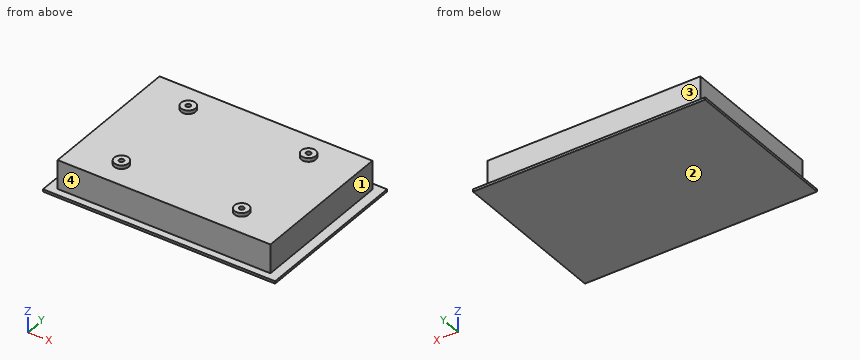
from build123d import *

# Parameters (mm, degrees)
SKETCH_1_W               = 193
SKETCH_1_H               = 134
EXTRUDE_1_DEPTH          = 2
SKETCH_2_W               = 177
SKETCH_2_H               = 122
EXTRUDE_2_DEPTH          = 24
CUT_EXTRUDE_1_DEPTH      = 10
CUT_EXTRUDE_1_DEPTH_BACK = 5
SKETCH_3_R               = 2
EXTRUDE_START            = 3
SKETCH_4_R               = 6
SKETCH_4_R_2             = 2
EXTRUDE_3_DEPTH          = 3


with BuildPart() as part:
    # 草图1 → 凸台-拉伸1 (new body)
    with BuildSketch(Plane.XY):
        Rectangle(SKETCH_1_W, SKETCH_1_H)
    extrude(amount=EXTRUDE_1_DEPTH)

    # 草图2 → 凸台-拉伸2 (add)
    with BuildSketch(Plane.XY.offset(2)):
        Rectangle(SKETCH_2_W, SKETCH_2_H)
    extrude(amount=EXTRUDE_2_DEPTH)

    # 草图3 → 切除-拉伸1 (cut, two sides: drawn at the far end of the back side and taken through both)
    with BuildSketch(Plane.XY.offset(26).offset(-CUT_EXTRUDE_1_DEPTH_BACK)):
        with Locations((-50, 40)):
            Circle(SKETCH_3_R)
        with Locations((-50, -40)):
            Circle(SKETCH_3_R)
        with Locations((50, -40)):
            Circle(SKETCH_3_R)
        with Locations((50, 40)):
            Circle(SKETCH_3_R)
    extrude(amount=CUT_EXTRUDE_1_DEPTH + CUT_EXTRUDE_1_DEPTH_BACK, mode=Mode.SUBTRACT)

    # 草图4 → 凸台-拉伸3 (add)
    # profile 1 of 4: a face of its own
    with BuildSketch(Plane.XY.offset(26).offset(EXTRUDE_START)):
        with Locations((-50, 40)):
            Circle(SKETCH_4_R)
        with Locations((-50, 40)):
            Circle(SKETCH_4_R_2, mode=Mode.SUBTRACT)
    # profile 2 of 4: a face of its own
    with BuildSketch(Plane.XY.offset(26).offset(EXTRUDE_START)):
        with Locations((-50, -40)):
            Circle(SKETCH_4_R)
        with Locations((-50, -40)):
            Circle(SKETCH_4_R_2, mode=Mode.SUBTRACT)
    # profile 3 of 4: a face of its own
    with BuildSketch(Plane.XY.offset(26).offset(EXTRUDE_START)):
        with Locations((50, -40)):
            Circle(SKETCH_4_R)
        with Locations((50, -40)):
            Circle(SKETCH_4_R_2, mode=Mode.SUBTRACT)
    # profile 4 of 4: a face of its own
    with BuildSketch(Plane.XY.offset(26).offset(EXTRUDE_START)):
        with Locations((50, 40)):
            Circle(SKETCH_4_R)
        with Locations((50, 40)):
            Circle(SKETCH_4_R_2, mode=Mode.SUBTRACT)
    extrude(amount=-EXTRUDE_3_DEPTH)


solid = part.part
Input: part model. Units: mm. Frame: model coordinates. Face numbers are marked on the shaded views. A direction names the side the tool comes from. Round coordinates to 2 decimals unless told otherwise and drop trailing zeros. Order: outer loops, then holes, each group sorted by start corner. A loop starts at its lowest first (then second) coordinate and runs counter-clockwise, first axis right, second up. Notation, with made-up numbers: (34, -34.5) - (53, -34.5) arc R24 cw to (53, -22.5) - close; hole circle Ø6 at (-16, 84.5). An arc over 180 degrees is marked (long way). Use a Markdown table: item, result.
1. First-contact query: pin 1 (2 mm diameter, centred on x = -50.5, y = -40, fed in from +Z); pin 2 (2 mm diameter, centred on y = -23.5, z = 22.5, fed in from -X); pin 3 (10 mm diameter, centred on y = -45.5, z = 22, fed in from +X). Flat tips, straight axial feed; report the tip coordinate or a pass-through.
Evaluation:
| item | result |
|---|---|
| pin 1 | z = 21 |
| pin 2 | x = -88.5 |
| pin 3 | x = 88.5 |
2. Material intervals for probe 1 along Y at (x, z) = (50, 22.55); probe 2 along Y at (x, z) = (50, 27.7); probe 3 along X at (y, z) = (39, 25.75), sorted ascending.
Evaluation:
| item | result |
|---|---|
| probe 1 | -61 to -42, -38 to 38, 42 to 61 |
| probe 2 | -46 to -42, -38 to -34, 34 to 38, 42 to 46 |
| probe 3 | -88.5 to -51.73, -48.27 to 48.27, 51.73 to 88.5 |
3. Access query for the marked faces 1, 2, 3 and 4. Directions: +Z, -Z, +X, -X, +Y, -Y. A direction counts if a zero-diameter tool reaches every point of the face in a straight line with its end or side. Return the directions, or none.
Evaluation:
| item | result |
|---|---|
| face 1 | +Z, +X, +Y, -Y |
| face 2 | -Z, +X, -X, +Y, -Y |
| face 3 | +Z, +X, -X, +Y |
| face 4 | +Z, +X, -X, -Y |
4. Section B-B on x = -18. Return the cut outline in (y, z).
Evaluation:
| item | result |
|---|---|
| outline | (-67, 0) - (67, 0) - (67, 2) - (61, 2) - (61, 26) - (-61, 26) - (-61, 2) - (-67, 2) - close |
5. Section C-C on x = -50. Return the cut outline in (y, z).
Evaluation:
| item | result |
|---|---|
| outline | (-67, 0) - (67, 0) - (67, 2) - (61, 2) - (61, 26) - (46, 26) - (46, 29) - (42, 29) - (42, 21) - (38, 21) - (38, 29) - (34, 29) - (34, 26) - (-34, 26) - (-34, 29) - (-38, 29) - (-38, 21) - (-42, 21) - (-42, 29) - (-46, 29) - (-46, 26) - (-61, 26) - (-61, 2) - (-67, 2) - close |
6. Section D-D on z = 6.75. Return the cut outline in (x, y), then the cut area to 3 significant figures.
Evaluation:
| item | result |
|---|---|
| outline | (-88.5, -61) - (88.5, -61) - (88.5, 61) - (-88.5, 61) - close |
| area | 21,600 mm^2 |
7. Section A-A on y = 40. Return the cut outline in (x, z), then the cut area to 3 significant figures.
Evaluation:
| item | result |
|---|---|
| outline | (-96.5, 0) - (96.5, 0) - (96.5, 2) - (88.5, 2) - (88.5, 26) - (56, 26) - (56, 29) - (52, 29) - (52, 21) - (48, 21) - (48, 29) - (44, 29) - (44, 26) - (-44, 26) - (-44, 29) - (-48, 29) - (-48, 21) - (-52, 21) - (-52, 29) - (-56, 29) - (-56, 26) - (-88.5, 26) - (-88.5, 2) - (-96.5, 2) - close |
| area | 4,640 mm^2 |
